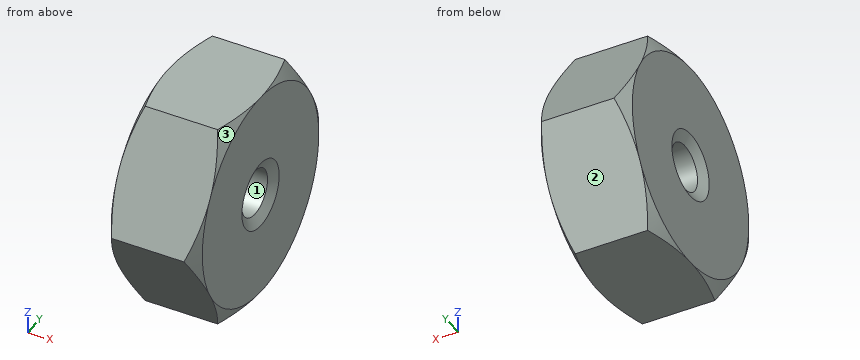
Autodesk Inventor part; units mm, degrees
ref_plane "Work Plane1" through (-6.3375, 0, 0) normal (0, -0.8660254, -0.5) x (1, 0, 0)
ref_plane "YZ Plane" through (0, 0, 0) normal (1, 0, 0) x (0, 1, 0)
ref_plane "XZ Plane" through (0, 0, 0) normal (0, 1, 0) x (-1, 0, 0)
sketch "Sketch1" plane through (0, 0, 0) normal (1, 0, 0) x (0, 1, 0)
  line L0 (-3.1754, 0) -> (-1.5877, 2.75)
  line L1 (-1.5877, 2.75) -> (1.5877, 2.75)
  line L2 (1.5877, 2.75) -> (3.1754, 0)
  line L3 (3.1754, 0) -> (1.5877, -2.75)
  line L4 (1.5877, -2.75) -> (-1.5877, -2.75)
  line L5 (-1.5877, -2.75) -> (-3.1754, 0)
  point P0 (0, 0)
  point P1 (0, 0)
  dimension "d0" = 6.3509
extrude "Body" add sketch "Sketch1" along normal blind 2.4
sketch "Sketch2" plane through (0, 0, 0) normal (0, 0, 1) x (1, 0, 0)
  line L0 (0, 1.5877) -> (0, 3.1754)
  line L1 (0, 3.1754) -> (2.4, 3.1754)
  line L2 (2.4, 1.5877) -> (2.4, 3.1754)
  line L3 (-0.16, 0) -> (0.96, 0)
  line L4 (0.2456, 3.1754) -> (0, 2.75)
  line L5 (2.1544, 3.1754) -> (2.4, 2.75)
  dimension "d3" = 30
  dimension "d4" = 30
  dimension "d5" = 5.5
  dimension "d6" = 5.5
revolve "Chamfer1" cut sketch "Sketch2" angle 360 about axis through (-10, 0, 0) along (1, 0, 0)
sketch "Sketch3" plane through (2.4, 0, 0) normal (1, 0, 0) x (0, 0, -1)
  arc A0 (-1.375, -2.3816) -> (1.375, -2.3816) centre (0, 0) ccw
hole "Thread" at (2.4, 0, 0) direction (-1, 0, 0) diameter 1.221 end through all
chamfer "Chamfer2" distance 0.2706 angle 30 1 edges at (2.4, 0, 0.6105) measured on face at (2.4, -2.0253, -0.0245)
chamfer "Chamfer3" distance 0.2706 angle 30 1 edges at (0, 0, 0.6105) measured on face at (0, -2.0253, -0.0245)
ref_plane "Work Plane1" through (-6.3375, 0, 0) normal (0, -0.8660254, -0.5) x (1, 0, 0)
equation "\"d0\" = 1.1547 * SW"
equation "\"d1\" = KOH"
equation "\"d3\" = ANG1"
equation "\"d4\" = ANG2"
equation "\"d5\" = SW0"
equation "\"d6\" = SW01"
equation "\"d8\" = -0.5 * GD1 + 0.5 * NND"
equation "\"d40\" = -0.5 * GD1 + 0.5 * NND"
equation "\"d10\" = -0.5 * GD1 + 0.5 * NND"
equation "\"d41\" = -0.5 * GD1 + 0.5 * NND"
equation "\"ANG1\" = 30deg"
equation "\"ANG2\" = 30deg"
equation "\"NND\" = 3"
equation "\"KOH\" = 2.4"
equation "\"SW\" = 5.5"
equation "\"SW0\" = SW"
equation "\"SW01\" = SW"
equation "\"GUL\" = 0.541266 * PTC"
equation "\"WFT\" = 0.4"
equation "\"THREADDIA\" = 3"
equation "\"TOA\" = 30deg"
equation "\"PTC\" = 0.5"
equation "\"E0\" = 1.155 * SW"
equation "\"GAL\" = 0.541266 * PTC"
properties part number "AS 1112 - M3  Type 5" material "Steel, Mild"
Geometry check sheet. Reference: the model listing, model coordinates, mm. Face numbers are marked on the shaded views. Round coordinates to 2 decimals unless told otherwise and drop trailing zeros. Order: outer loops, then holes, each group sorted by start corner. A loop starts at its lowest first (then second) coordinate and runs counter-clockwise, first axis right, second up. Notation, with made-up numbers: M -33,-15 L -10,-15 A34 cw -10,23 Z; hole C -8,80.5 d4. An arc over 180 degrees is marked long. Answer in a Markdown table with one row per item. Add a question column.
Item 1: Material ranges on L1, parallel to Z at x = 1.35, y = 0; L2, parallel to Z at x = 0.2, y = -0.5; L3, parallel to Y at x = 1.7, z = -2.3, recorded low to high. Write a range as [from, to].
Item 2: Sectioned sample at A-A, the plane x = 1.7. Enter the section's corners in (y, z).
Item 3: Depth check by flat-ended pin: pin 1 Ø1.1 at (y, z) = (0, 0) entering from -X. Enter the tip coordinate at first touch or a pass-through.
Item 4: Draft check along Y on the marked faces 1, 2 and 3. Enter one of: released by +Y, released by -Y, zero draft, split by the parting line, or undercut.
Filled in:
| question | item | result |
|---|---|---|
| 1 | L1 | z = [-2.75, -0.61], [0.61, 2.75] |
| 1 | L2 | z = [-2.75, -0.35], [0.35, 2.75] |
| 1 | L3 | y = [-1.85, 1.85] |
| 2 | outline | M -3.18,0 L -1.59,-2.75 L 1.59,-2.75 L 3.18,0 L 1.59,2.75 L -1.59,2.75 Z; hole C 0,0 d1.22 |
| 3 | pin 1 | passes through |
| 4 | face 1 | undercut |
| 4 | face 2 | released by +Y |
| 4 | face 3 | released by -Y |
